```python
from build123d import *

# Parameters (mm, degrees)
SKETCH1_R           = 2.5
SKETCH1_R_2         = 0.6
SKETCH1_R_3         = 1
BOSS_EXTRUDE1_DEPTH = 2.5
SKETCH2_R           = 1
CUT_EXTRUDE1_DEPTH  = 46.745081512


with BuildPart() as part:
    # Sketch1 → Boss-Extrude1 (new body)
    # profile 1 of 3: a face of its own
    with BuildSketch(Plane(origin=(0, 0, 0), x_dir=(1, 0, 0), z_dir=(0, 1, 0))):
        Circle(SKETCH1_R)
        with Locations(Location((0, 0, 0), (0, 0, 270))):
            Circle(SKETCH1_R_2, mode=Mode.SUBTRACT)
    # profile 2 of 3: a face of its own
    with BuildSketch(Plane(origin=(0, 0, 0), x_dir=(1, 0, 0), z_dir=(0, 1, 0))):
        with BuildLine():
            ThreePointArc((-1.180555556, 2.203698841), (1.284252917, 2.144922946), (2.5, 0))
            ThreePointArc((2.5, 0), (2.144922946, -1.284252917), (1.180555556, -2.203698841))
            ThreePointArc((1.180555556, -2.203698841), (21.25, 2.833420868), (41.319444444, -2.203698841))
            ThreePointArc((41.319444444, -2.203698841), (40.296301159, 1.180555556), (43.680555556, 2.203698841))
            ThreePointArc((43.680555556, 2.203698841), (21.25, 7.833420868), (-1.180555556, 2.203698841))
        make_face()
    # profile 3 of 3: a face of its own
    with BuildSketch(Plane(origin=(0, 0, 0), x_dir=(1, 0, 0), z_dir=(0, 1, 0))):
        with Locations((42.5, 0)):
            Circle(SKETCH1_R)
        with Locations(Location((42.5, 0, 0), (0, 0, 270))):
            Circle(SKETCH1_R_3, mode=Mode.SUBTRACT)
    extrude(amount=BOSS_EXTRUDE1_DEPTH)

    # Sketch2 → Cut-Extrude1 (cut, through all)
    with BuildSketch(Plane(origin=(0, 2.5, 0), x_dir=(1, 0, 0), z_dir=(0, 1, 0))):
        with Locations(Location((12.25, 4.424236239, 0), (0, 0, 270))):
            Circle(SKETCH2_R)
        with Locations(Location((30.25, 4.424236239, 0), (0, 0, 270))):
            Circle(SKETCH2_R)
    extrude(amount=-CUT_EXTRUDE1_DEPTH, mode=Mode.SUBTRACT)


solid = part.part
```
Model file for the job. Use its own axes, mm. Give positions to 0.01 mm unless a question says otherwise; leave off trailing zeros. Loops run counter-clockwise (first coordinate to the right, second up) from the corner with the lowest first, then second, coordinate; pieces in that order, holes last. Notation, with made-up numbers: (-14.75, 66) -> (-1.75, 66) arc R15 cw to (-1.75, 75) -> close; hole circle Ø6 at (50.5, 31.5). An arc over 180 degrees is marked (long way). Use CSV: the item, a comma, the result in double quotes. Start each with the question number.
1) Slice it at A-A on y = 1.2. Give the cut face in (x, z).
2) Mould opens along X. For faces 1 (the cylindrical face through (11.274, 1.268, -4.641)), 2 (the flat face through (21, 0, -4)), 3 (the cylindrical face through (0.506, 1.232, 0.323)), 4 (the cylindrical face through (21.577, 1.232, -7.832)) say: released by +X, released by -X, zero draft, split by the parting line, or undercut.
3) Flat gauge pins, fed straight in: pin 1 Ø1 at (y, z) = (2, -2) entering from +X; pin 2 Ø1 at (x, z) = (0, 0) entering from +Y. Where does each tip first touch, or does it go through?
4) Slice it at B-B on z = 1.5. Give the cut face in (x, y).
5) Wall check: line 1 (X direction, y = 0.5, z = -3.75); line 2 (X direction, y = 1.65, z = 2); line 3 (Z direction, x = 12, y = 0.7). Give the ranges that are in metal, low to high.
6) Slice it at C-C on x = 12.25. Give the cut face in (y, z).
7) Slice it at D-D on x = 33.5. Give the cut face in (y, z).
Computed values:
1,outline,"(-1.18, -2.2) arc R47.5 ccw to (43.68, -2.2) arc R2.5 ccw to (41.32, 2.2) arc R42.5 cw to (1.18, 2.2) arc R2.5 ccw to start; hole circle Ø1.2 at (0, 0); hole circle Ø2 at (12.25, -4.42); hole circle Ø2 at (30.25, -4.42); hole circle Ø2 at (42.5, 0)"
2,face 1,"undercut"
2,face 2,"zero draft"
2,face 3,"undercut"
2,face 4,"split by the parting line"
3,pin 1,"stops at x = 44.5"
3,pin 2,"passes through"
4,outline,"(-2, 0) -> (2.55, 0) -> (2.55, 2.5) -> (-2, 2.5) -> close; (39.95, 0) -> (44.5, 0) -> (44.5, 2.5) -> (39.95, 2.5) -> close"
5,line 1,"x = 1.98 to 11.51, 12.99 to 29.51, 30.99 to 40.52"
5,line 2,"x = -1.5 to 1.57, 40.93 to 44"
5,line 3,"z = -6.92 to -5.39, -3.46 to -1.81"
6,outline,"(0, -6.97) -> (2.5, -6.97) -> (2.5, -5.42) -> (0, -5.42) -> close; (0, -3.42) -> (2.5, -3.42) -> (2.5, -1.87) -> (0, -1.87) -> close"
7,outline,"(0, -6.23) -> (2.5, -6.23) -> (2.5, -1.03) -> (0, -1.03) -> close"
